```python
from build123d import *

# Parameters (mm, degrees)
F1_DEPTH = 7.9375
F4_DEPTH = 25.4
F5_DEPTH = 25.4


with BuildPart() as f1:
    # F0 (on Right) → F1 (new body, symmetric)
    with BuildSketch(Plane.YZ):
        Polygon((4.7625, 0), (4.7625, 50.8), (-1.5875, 50.8), (-1.5875, 0), (-1.5875, -69.85), (4.7625, -69.85), (42.8625, -69.85), (42.8625, -63.5), (4.7625, -63.5), (4.7625, -6.35), (42.8625, -6.35), (42.8625, 0), align=None)
    extrude(amount=F1_DEPTH, both=True)

    # F3 (on face) → F4 (cut)
    with BuildSketch(Plane.XZ.offset(1.5875)):
        with BuildLine():
            ThreePointArc((0, 22.225), (2.245064, 23.154936), (3.175, 25.4))
            ThreePointArc((3.175, 25.4), (-2.245064, 27.645064), (0, 22.225))
        make_face()
    extrude(amount=-F4_DEPTH, mode=Mode.SUBTRACT)

    # F2 (on face) → F5 (cut)
    with BuildSketch(Plane.XY.offset(-63.5)):
        with BuildLine():
            ThreePointArc((2.38125, 30.1625), (-1.683798, 31.846298), (0, 27.78125))
            ThreePointArc((0, 27.78125), (1.683798, 28.478702), (2.38125, 30.1625))
        make_face()
    extrude(amount=-F5_DEPTH, mode=Mode.SUBTRACT)


solid = f1.part
```
Source: CAD feature listing. Evaluate the final solid. Frame: model axes, mm. A direction names the side the tool comes from. Round coordinates to 2 decimals unless told otherwise and drop trailing zeros. Loops run counter-clockwise (first coordinate to the right, second up) from the corner with the lowest first, then second, coordinate; pieces in that order, holes last. Notation, with made-up numbers: M -30,83.5 L -24,83.5 A35 ccw -24,122.5 Z; hole C 80,-2 d5. An arc over 180 degrees is marked long. Use a Markdown table: item, result. Add a question column.
1. Cut plane A-A, the plane y = 6. Output: boundary loops of the cut face in (x, z), and give its area (3 significant figures).
2. Contact query for flat-ended pins moving along their axis: pin 1 (5 mm diameter, centred on x = 4.5, z = 30, fed in from +Y); pin 2 (10 mm diameter, centred on y = 19.5, z = -13, fed in from +X); pin 3 (7.5 mm diameter, centred on x = 0, y = 30.16, fed in from +Z). Output: stop coordinate, or through.
3. Set-up query: faces 1 (the flat face through (0, 24, 0)), 2 (the flat face through (-7.938, 4, -18)), 3 (the flat face through (0, 24, -6.35)). Return all of +Z, -Z, +X, -X, +Y, -Y with unobstructed straight access to the full face (end or side cutting, diameter ignored); none if empty.
4. Cut plane B-B, the plane x = 5. Output: boundary loops of the cut face in (y, z).
5. Ray query, line 1 along X through (y, z) = (1, 25); line 2 along Z through (x, y) = (0, 3.25) (3 decimals); line 3 along X through (y, z) = (0.5, 25.4) (1 decimal). Return the intervals inside material, ascending. Write a range as [from, to].
6. Pull-direction query (Z, two-part tool) for faces 4 (the flat face through (0, 24, -63.5)), 5 (the flat face through (0, 2, 50.8)), 6 (the flat face through (4, 4.762, 25)), 7 (the flat face through (0, 4.762, -35)); classes: +Z half, -Z half, draft (parallel to the pull), parting line (faces both ways), or undercut.
7. Cut plane C-C, the plane y = 29. Output: boundary loops of the cut face in (x, z), and give its area (3 significant figures).
8. Cut plane D-D, the plane z = -44.5. Output: boundary loops of the cut face in (x, y).
Solution:
| question | item | result |
|---|---|---|
| 1 | outline | M -7.94,-69.85 L 7.94,-69.85 L 7.94,-63.5 L -7.94,-63.5 Z; M -7.94,-6.35 L 7.94,-6.35 L 7.94,0 L -7.94,0 Z |
| 1 | area | 202 mm2 |
| 2 | pin 1 | stops at y = 4.76 |
| 2 | pin 2 | passes through |
| 2 | pin 3 | stops at z = 0 |
| 3 | face 1 | +Z, +X, -X, +Y |
| 3 | face 2 | +Z, -Z, -X, +Y, -Y |
| 3 | face 3 | +X, -X, +Y |
| 4 | outline | M -1.59,-69.85 L 42.86,-69.85 L 42.86,-63.5 L 4.76,-63.5 L 4.76,-6.35 L 42.86,-6.35 L 42.86,0 L 4.76,0 L 4.76,50.8 L -1.59,50.8 Z |
| 5 | line 1 | x = [-7.94, -3.15], [3.15, 7.94] |
| 5 | line 2 | z = [-69.85, 22.225], [28.575, 50.8] |
| 5 | line 3 | x = [-7.9, -3.2], [3.2, 7.9] |
| 6 | face 4 | undercut |
| 6 | face 5 | +Z half |
| 6 | face 6 | draft |
| 6 | face 7 | undercut |
| 7 | outline | M -7.94,-69.85 L -2.08,-69.85 L -2.08,-63.5 L -7.94,-63.5 Z; M -7.94,-6.35 L 7.94,-6.35 L 7.94,0 L -7.94,0 Z; M 2.08,-69.85 L 7.94,-69.85 L 7.94,-63.5 L 2.08,-63.5 Z |
| 7 | area | 175 mm2 |
| 8 | outline | M -7.94,-1.59 L 7.94,-1.59 L 7.94,4.76 L -7.94,4.76 Z |
